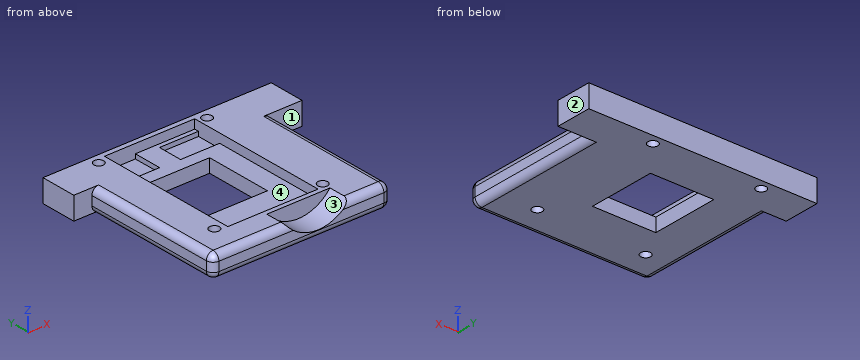
from build123d import *

# Parameters (mm, degrees)
SKETCH1_W               = 19.78
SKETCH1_H               = 22
BOSS_EXTRUDE1_DEPTH     = 2.5
SKETCH2_R               = 0.55
CUT_EXTRUDE1_DEPTH      = 2.5
SKETCH3_W               = 7.014228963
SKETCH3_H               = 7.519558389
CUT_EXTRUDE2_DEPTH      = 2.5
SKETCH4_W               = 10
SKETCH4_H               = 16
CUT_EXTRUDE3_DEPTH      = 1
SKETCH5_W               = 4.325292028
SKETCH5_H               = 2.74046394
SKETCH5_W_2             = 3.425085756
SKETCH5_H_2             = 3.145892333
CUT_EXTRUDE4_DEPTH      = 0.5
SKETCH6_R               = 4.45
CUT_EXTRUDE5_DEPTH      = 1.5
CUT_EXTRUDE5_DEPTH_BACK = 1.1
SKETCH7_W               = 19.78
SKETCH7_H               = 2.5
CUT_EXTRUDE6_DEPTH      = 2.4
SKETCH8_W               = 3.5
SKETCH8_H               = 4
SKETCH8_W_2             = 2
BOSS_EXTRUDE2_DEPTH     = 2.5
FILLET1_R               = 0.75


with BuildPart() as part:
    # Sketch1 → Boss-Extrude1 (new body)
    with BuildSketch(Plane.XY):
        with Locations((16.80685162, -7.939657117)):
            Rectangle(SKETCH1_W, SKETCH1_H)
    extrude(amount=BOSS_EXTRUDE1_DEPTH)

    # Sketch2 → Cut-Extrude1 (cut)
    with BuildSketch(Plane.XY.offset(2.5)):
        with Locations((22.156215749, -0.440049881)):
            Circle(SKETCH2_R)
        with Locations((22.156215749, -15.440049881)):
            Circle(SKETCH2_R)
        with Locations((10.156215749, -15.440049881)):
            Circle(SKETCH2_R)
        with Locations((10.156215749, -0.440049881)):
            Circle(SKETCH2_R)
    extrude(amount=-CUT_EXTRUDE1_DEPTH, mode=Mode.SUBTRACT)

    # Sketch3 → Cut-Extrude2 (cut)
    with BuildSketch(Plane.XY.offset(2.5)):
        with Locations((15.488045681, -8.221060457)):
            Rectangle(SKETCH3_W, SKETCH3_H)
    extrude(amount=-CUT_EXTRUDE2_DEPTH, mode=Mode.SUBTRACT)

    # Sketch4 → Cut-Extrude3 (cut)
    with BuildSketch(Plane.XY.offset(2.5)):
        with Locations((16.25685162, -7.889657117)):
            Rectangle(SKETCH4_W, SKETCH4_H)
    extrude(amount=-CUT_EXTRUDE3_DEPTH, mode=Mode.SUBTRACT)

    # Sketch5 → Cut-Extrude4 (cut)
    with BuildSketch(Plane.XY.offset(1.5)):
        with Locations((19.094205606, -1.748569373)):
            Rectangle(SKETCH5_W, SKETCH5_H)
        with Locations((12.969394498, -1.462603284)):
            Rectangle(SKETCH5_W_2, SKETCH5_H_2)
    extrude(amount=-CUT_EXTRUDE4_DEPTH, mode=Mode.SUBTRACT)

    # Sketch6 → Cut-Extrude5 (cut, two sides)
    with BuildSketch(Plane.XZ.offset(17.489657117)) as cut_extrude5_sk:
        with Locations((18.65685162, 5.25)):
            Circle(SKETCH6_R)
    extrude(amount=CUT_EXTRUDE5_DEPTH, mode=Mode.SUBTRACT)
    extrude(cut_extrude5_sk.sketch, amount=-CUT_EXTRUDE5_DEPTH_BACK, mode=Mode.SUBTRACT)

    # Sketch7 → Cut-Extrude6 (cut)
    with BuildSketch(Plane(origin=(0, 3.060342883, 0), x_dir=(1, 0, 0), z_dir=(0, 1, 0))):
        with Locations((16.80685162, -1.25)):
            Rectangle(SKETCH7_W, SKETCH7_H)
    extrude(amount=-CUT_EXTRUDE6_DEPTH, mode=Mode.SUBTRACT)

    # Sketch8 → Boss-Extrude2 (add)
    with BuildSketch(Plane.XY.offset(2.5)):
        with Locations((28.44685162, -1.339657117)):
            Rectangle(SKETCH8_W, SKETCH8_H)
        with Locations((5.91685162, -1.339657117)):
            Rectangle(SKETCH8_W_2, SKETCH8_H)
    extrude(amount=-BOSS_EXTRUDE2_DEPTH)

    # Fillet1
    fillet1_edges = [part.edges().sort_by_distance(p)[0] for p in [
        (6.91685162, -11.139657117, 0),
        (6.91685162, -11.139657117, 2.5),
        (11.037566052, -18.939657117, 2.5),
        (26.69685162, -11.139657117, 2.5),
        (16.80685162, -18.939657117, 0),
        (26.69685162, -11.139657117, 0),
        (26.69685162, -18.939657117, 1.25),
        (6.91685162, -18.939657117, 1.25),
        (24.426137189, -18.939657117, 2.5),
    ]]
    fillet(fillet1_edges, radius=FILLET1_R)


solid = part.part
CAD build for the part. Positions are in the model's coordinates, mm. Face numbers are marked on the shaded views. Give positions to 0.01 mm unless a question says otherwise; leave off trailing zeros. Order: outer loops, then holes, each group sorted by start corner. A loop starts at its lowest first (then second) coordinate and runs counter-clockwise, first axis right, second up. Notation, with made-up numbers: (-37.5, -16.5) - (5.5, -16.5) arc R19 ccw to (5.5, 2.5) - close; hole circle Ø5 at (57, -25.5). An arc over 180 degrees is marked (long way). Write each question's results on one line, items separated by ' | '.
1. Saw through at B-B on y = -10.25. List the corners of the cut face in (x, z), and give its area (3 significant figures).
Calculated:
outline: (6.92, 0.75) arc R0.75 ccw to (7.67, 0) - (11.98, 0) - (11.98, 1.5) - (11.26, 1.5) - (11.26, 2.5) - (7.67, 2.5) arc R0.75 ccw to (6.92, 1.75) - close; (19, 0) - (25.95, 0) arc R0.75 ccw to (26.7, 0.75) - (26.7, 1.75) arc R0.75 ccw to (25.95, 2.5) - (21.26, 2.5) - (21.26, 1.5) - (19, 1.5) - close | area: 28.4 mm2
2. Saw through at D-D on z = 2.15. List the corners of the cut face in (x, y).
Calculated:
outline: (4.92, -3.34) - (7.03, -3.34) - (7.03, -18.19) arc R0.63 ccw to (7.67, -18.82) - (15.46, -18.82) - (15.46, -16.39) - (21.85, -16.39) - (21.85, -18.82) - (25.95, -18.82) arc R0.63 ccw to (26.58, -18.19) - (26.58, -3.34) - (30.2, -3.34) - (30.2, 0.66) - (4.92, 0.66) - close; hole circle Ø1.1 at (10.16, -15.44); hole circle Ø1.1 at (10.16, -0.44); hole (11.26, -15.89) - (21.26, -15.89) - (21.26, 0.11) - (11.26, 0.11) - close; hole circle Ø1.1 at (22.16, -15.44); hole circle Ø1.1 at (22.16, -0.44)
3. Saw through at C-C on y = -2.5. List the corners of the cut face in (x, z), and give its area (3 significant figures).
Calculated:
outline: (4.92, 0) - (30.2, 0) - (30.2, 2.5) - (21.26, 2.5) - (21.26, 1) - (16.93, 1) - (16.93, 1.5) - (14.68, 1.5) - (14.68, 1) - (11.26, 1) - (11.26, 2.5) - (4.92, 2.5) - close | area: 49.3 mm2
4. Pull direction X, two halves, no side cores. Call the marked faces 1, 2, 3 and 4: released by +X, released by -X, zero draft, split by the parting line, or undercut.
Calculated:
face 1: zero draft | face 2: released by +X | face 3: undercut | face 4: undercut
5. Probe L1, parallel to Y at x = 14.5, z = 1.35; L2, parallel to X at y = -5.5, z = 0.75; L3, parallel to Y at x = 19.75, z = 1.4. List the from-to ranges inside material, lowest first. Write a range as from..to.
Calculated:
L1: y = -18.94..-11.98, -4.46..-3.04, 0.11..0.66 | L2: x = 6.92..11.98, 19..26.7 | L3: y = -16.39..-3.12, -0.38..0.66
6. Saw through at A-A on x = 13.25. List the corners of the cut face in (y, z).
Calculated:
outline: (-18.94, 0.75) arc R0.75 ccw to (-18.19, 0) - (-11.98, 0) - (-11.98, 1.5) - (-15.89, 1.5) - (-15.89, 2.5) - (-18.19, 2.5) arc R0.75 ccw to (-18.94, 1.75) - close; (-4.46, 0) - (0.66, 0) - (0.66, 2.5) - (0.11, 2.5) - (0.11, 1) - (-3.04, 1) - (-3.04, 1.5) - (-4.46, 1.5) - close
7. Pin check, flat tips, straight feed: pin 1 (1.1 mm diameter, centred on y = -11.5, z = 1, fed in from +X); pin 2 (1.5 mm diameter, centred on y = -17, z = 1, fed in from -X); pin 3 (0.7 mm diameter, centred on x = 22.16, y = -0.44, fed in from -Z); pin 4 (0.6 mm diameter, centred on x = 19, z = 1.5, fed in from -Y). Stop position of each tip, or through.
Calculated:
pin 1: stops at x = 26.7 | pin 2: stops at x = 6.92 | pin 3: passes through | pin 4: stops at y = -16.39
